```python
from build123d import *

# Parameters (mm, degrees)
F1_DEPTH = 10
F2_R     = 2
F3_DEPTH = 10.001
F4_R     = 2
F5_DEPTH = 15.530304


with BuildPart() as f1:
    # F0 (on Top) → F1 (new body)
    with BuildSketch(Plane.XY):
        with BuildLine():
            ThreePointArc((-15.4, 0), (0, 15.4), (15.4, 0))
            Line((15.4, 0), (19.4, 0))
            Line((19.4, 0), (34.4, 0))
            ThreePointArc((34.4, 0), (37.935534, -1.464466), (39.4, -5))
            Line((39.4, -5), (39.4, -6))
            Line((39.4, -6), (62.642914, 34.257907))
            Line((62.642914, 34.257907), (64.642914, 37.722009))
            Line((64.642914, 37.722009), (68.642914, 44.650212))
            Line((68.642914, 44.650212), (70.642914, 48.114314))
            Line((70.642914, 48.114314), (88.473701, 78.998144))
            Line((88.473701, 78.998144), (90.473701, 82.462245))
            Line((90.473701, 82.462245), (94.473701, 89.390449))
            Line((94.473701, 89.390449), (96.473701, 92.85455))
            Line((96.473701, 92.85455), (118.730127, 131.403811))
            Line((118.730127, 131.403811), (116.132051, 132.903811))
            Line((116.132051, 132.903811), (114.4, 133.903811))
            Line((114.4, 133.903811), (39.97735, 5))
            ThreePointArc((39.97735, 5), (39.245299, 4.267949), (38.245299, 4))
            Line((38.245299, 4), (30.864102, 4))
            ThreePointArc((30.864102, 4), (29.132051, 5), (29.132051, 7))
            Line((29.132051, 7), (30.592345, 9.529304))
            Line((30.592345, 9.529304), (16.898295, 9.529304))
            ThreePointArc((16.898295, 9.529304), (-2.219193, 19.272654), (-18.621883, 5.439252))
            ThreePointArc((-18.621883, 5.439252), (-19.341977, 4.399766), (-20.541665, 4))
            Line((-20.541665, 4), (-31.4, 4))
            Line((-31.4, 4), (-31.4, 0))
            Line((-31.4, 0), (-19.4, 0))
            Line((-19.4, 0), (-15.4, 0))
        make_face()
        Polygon((64.642914, 37.722009), (62.642914, 34.257907), (73.035219, 28.257907), (81.035219, 42.114314), (70.642914, 48.114314), (68.642914, 44.650212), (75.571117, 40.650212), (71.571117, 33.722009), align=None)
        Polygon((90.473701, 82.462245), (88.473701, 78.998144), (98.866006, 72.998144), (106.866006, 86.85455), (96.473701, 92.85455), (94.473701, 89.390449), (101.401904, 85.390449), (97.401904, 78.462245), align=None)
    extrude(amount=F1_DEPTH)

    # F2 (on face) → F3 (cut, through all)
    with BuildSketch(Plane(origin=(0, 4, 0), x_dir=(-1, 0, 0), z_dir=(0, 1, 0))):
        with Locations((25.970832, 5)):
            Circle(F2_R)
    extrude(amount=-F3_DEPTH, mode=Mode.SUBTRACT)

    # F4 (on face) → F5 (cut, through all)
    with BuildSketch(Plane(origin=(0, 9.529304, 0), x_dir=(-1, 0, 0), z_dir=(0, 1, 0))):
        with Locations((-23.898295, 5)):
            Circle(F4_R)
    extrude(amount=-F5_DEPTH, mode=Mode.SUBTRACT)


solid = f1.part
```
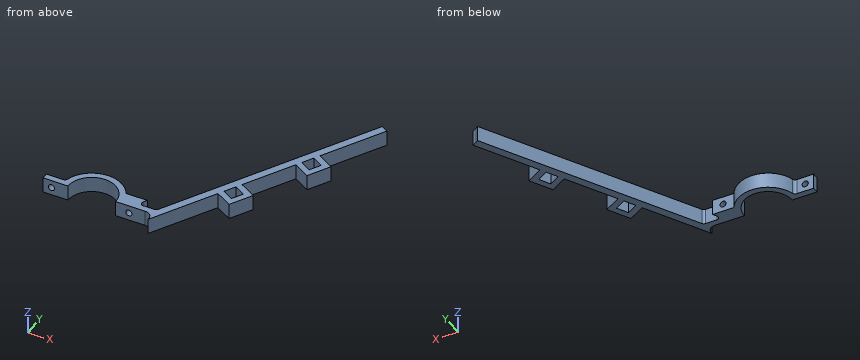
Could you check a few things on this model? Use its own coordinates, in mm. Give positions to 0.01 mm unless a question says otherwise; leave off trailing zeros. Order: outer loops, then holes, each group sorted by start corner. A loop starts at its lowest first (then second) coordinate and runs counter-clockwise, first axis right, second up.
Q1. Suppose I cut it at B-B, the plane x = 0. Write out the boundary of the cut face in (y, z).
Q2. Suppose I cut it at C-C, the plane y = 54. Write out the boundary of the cut face in (x, z).
Q3. I'm going to push flat-ended pins straight in: P1, Ø3, axis at y = 87, z = 3.5, coming from the +X side; P2, Ø3, axis at x = 15.5, z = 5.5, coming from the -Y side; P3, Ø1, axis at x = 81, z = 7, coming from the +Y side. Where does each tip first touch, or does it pass through?
Q4. Suppose I cut it at A-A, the plane z = 1.5. Count the separate pieces of the cut face and the enclosed holes in it, and give its area (3 significant figures).
Q5. If I drill on line 1 along X through (y, z) = (6, 7.25); line 2 along Y through (x, z) = (99.5, 9); line 3 along Y through (x, z) = (-22, 1.5), over which ranges is the centre line in solid material (lowest first)?
Solution:
1. outline: (15.4, 0) - (19.4, 0) - (19.4, 10) - (15.4, 10) - close
2. outline: (68.27, 0) - (74.04, 0) - (74.04, 10) - (68.27, 10) - close
3. P1: stops at x = 106.87
3. P2: stops at y = 0
3. P3: stops at y = 76.92
4. separate pieces: 1
4. enclosed holes: 2
4. area: 1,440 mm2
5. line 1: x = -18.45 to -14.18, 14.18 to 28.86, 40.55 to 46.33
5. line 2: y = 74.1 to 82.1, 86.49 to 91.11, 98.1 to 108.1
5. line 3: y = 0 to 4
